Print and shaded views of the part. All mm, measured from the part's lowest x, y and z. A direction names the side the tool comes from. Coordinates: 2 decimals unless noted, no trailing zeros. Loops run counter-clockwise (first coordinate to the right, second up) from the corner with the lowest first, then second, coordinate; pieces in that order, holes last. Notation, with made-up numbers: M 55.5,34 L 102.5,34 A22 cw 102.5,55 Z; hole C 51.25,65.25 d11. An arc over 180 degrees is marked long. Use a Markdown table: item, result. Add a question column.
1) Pull direction X, two halves, no side cores. Call the marked faces 6 and 7: released by +X, released by -X, zero draft, split by the parting line, or undercut.
2) Band-saw the part on B-B (z = 26.5). List the corners of the cut face in (x, y), plus the area to 3 significant figures.
3) Tool access for the marked faces 1, 2, 3, 4 and 5: list every direction of +Z, -Z, +X, -X, +Y, -Y with a clear straight run to the whole face (end or side of a thin tool).
4) Band-saw the part on C-C (y = 288). List the corners of the cut face in (x, z).
5) Pin check, flat tips, straight feed: pin 1 Ø9.5 at (y, z) = (8.5, 24.5) entering from +X; pin 2 Ø1 at (x, y) = (802.5, 161.5) entering from +Z; pin 3 Ø9.5 at (y, z) = (3.5, 19) entering from -X. Stop position of each tip, or through.
6) Wall check: probe 1 along X at (y, z) = (506.5, 105); probe 2 along Y at (x, z) = (237, 139); probe 3 along Z at (x, y) = (562, 192). Give the ranges that are in metal, low to high. Write a range as from..to.
7) Band-saw the part on A-A (x = 755). List the corners of the cut face in (y, z), plus the area to 3 significant figures.
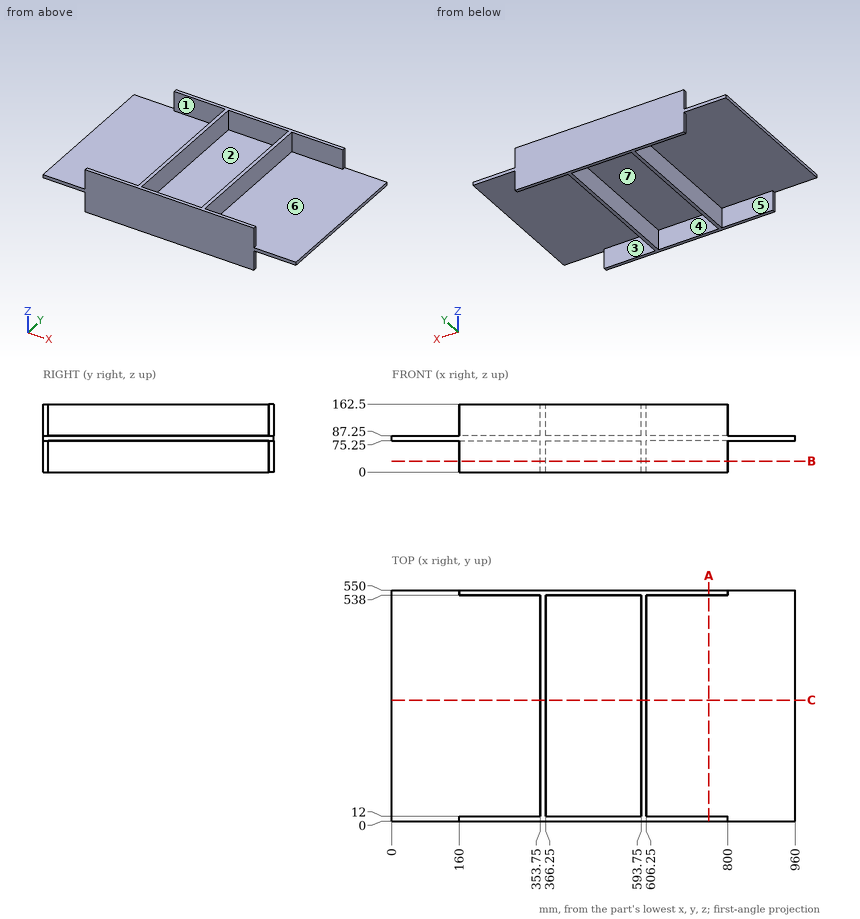
Entries:
| question | item | result |
|---|---|---|
| 1 | face 6 | zero draft |
| 1 | face 7 | undercut |
| 2 | outline | M 160,0 L 800,0 L 800,12 L 606.25,12 L 606.25,538 L 800,538 L 800,550 L 160,550 L 160,538 L 353.75,538 L 353.75,12 L 160,12 Z; hole M 366.25,12 L 593.75,12 L 593.75,538 L 366.25,538 Z |
| 2 | area | 28,500 mm2 |
| 3 | face 1 | +Z, -X |
| 3 | face 2 | +Z |
| 3 | face 3 | -Z, +X |
| 3 | face 4 | -Z |
| 3 | face 5 | -Z, -X |
| 4 | outline | M 0,75.25 L 353.75,75.25 L 353.75,0 L 366.25,0 L 366.25,75.25 L 593.75,75.25 L 593.75,0 L 606.25,0 L 606.25,75.25 L 960,75.25 L 960,87.25 L 606.25,87.25 L 606.25,162.5 L 593.75,162.5 L 593.75,87.25 L 366.25,87.25 L 366.25,162.5 L 353.75,162.5 L 353.75,87.25 L 0,87.25 Z |
| 5 | pin 1 | x = 800 |
| 5 | pin 2 | z = 87.25 |
| 5 | pin 3 | x = 160 |
| 6 | probe 1 | 353.75..366.25, 593.75..606.25 |
| 6 | probe 2 | 0..12, 538..550 |
| 6 | probe 3 | 75.25..87.25 |
| 7 | outline | M 0,0 L 12,0 L 12,75.25 L 538,75.25 L 538,0 L 550,0 L 550,162.5 L 538,162.5 L 538,87.25 L 12,87.25 L 12,162.5 L 0,162.5 Z |
| 7 | area | 10,200 mm2 |
